Verification items for the finished model (mm, model axes). Give positions to 0.01 mm unless a question says otherwise; leave off trailing zeros. Write each loop counter-clockwise with the first axis right and the second up, starting at its lowest first coordinate (ties: lowest second). Pieces come first, ordered by that corner, then holes. Notation, with made-up numbers: M -15,-1.5 L 10,-1.5 A29 cw 10,21.5 Z; hole C 81.25,31.5 d5. An arc over 180 degrees is marked long. Answer as a JSON object with one key per item and string values.
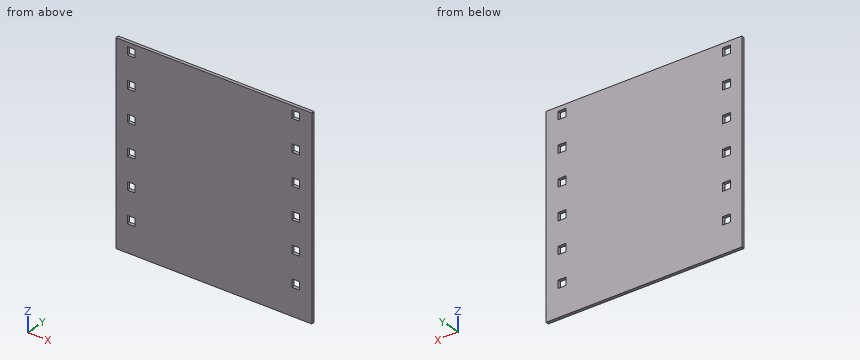
Autodesk Inventor part; units mm, degrees
ref_plane "YZ Plane" through (0, 0, 0) normal (1, 0, 0) x (0, 1, 0)
ref_plane "XZ Plane" through (0, 0, 0) normal (0, 1, 0) x (-1, 0, 0)
ref_plane "XY Plane" through (0, 0, 0) normal (0, 0, 1) x (1, 0, 0)
sketch "Эскиз1" plane through (0, 0, 0) normal (0, 1, 0) x (-1, 0, 0)
  line L0 (125, 125) -> (-125, 125)
  line L1 (-125, 125) -> (-125, -125)
  line L2 (-125, -125) -> (125, -125)
  line L3 (125, -125) -> (125, 125)
  line L4 (125, 125) -> (-125, -125) construction
  line L5 (-125, 125) -> (125, -125) construction
  point P0 (0, 0)
  dimension "d0" = 250
  dimension "d1" = 250
extrude "Выдавливание1" add sketch "Эскиз1" along normal blind 4
sketch "Эскиз2" plane through (0, 0, 0) normal (0, -1, 0) x (1, 0, 0)
  line L0 (-110.387511, 109.588885) -> (-110.387511, 119.588885)
  line L1 (-100.387511, 109.588885) -> (-110.387511, 109.588885)
  line L2 (-100.387511, 119.588885) -> (-100.387511, 109.588885)
  line L3 (-110.387511, 119.588885) -> (-100.387511, 119.588885)
  line L4 (-110.387511, 29.588885) -> (-110.387511, 39.588885)
  line L5 (-100.387511, 29.588885) -> (-110.387511, 29.588885)
  line L6 (-100.387511, 39.588885) -> (-100.387511, 29.588885)
  line L7 (-110.387511, 39.588885) -> (-100.387511, 39.588885)
  line L8 (-110.387511, -10.411115) -> (-110.387511, -0.411115)
  line L9 (-100.387511, -10.411115) -> (-110.387511, -10.411115)
  line L10 (-100.387511, -0.411115) -> (-100.387511, -10.411115)
  line L11 (-110.387511, -0.411115) -> (-100.387511, -0.411115)
  line L12 (125, 125) -> (125, -125)
  line L13 (-125, 125) -> (125, 125)
  line L14 (-125, -125) -> (-125, 125)
  line L15 (125, -125) -> (-125, -125)
  line L16 (109.612489, 109.588885) -> (109.612489, 119.588885)
  line L17 (109.612489, 119.588885) -> (99.612489, 119.588885)
  line L18 (99.612489, 119.588885) -> (99.612489, 109.588885)
  line L19 (99.612489, 109.588885) -> (109.612489, 109.588885)
  line L20 (109.612489, 29.588885) -> (109.612489, 39.588885)
  line L21 (109.612489, 39.588885) -> (99.612489, 39.588885)
  line L22 (99.612489, 39.588885) -> (99.612489, 29.588885)
  line L23 (99.612489, 29.588885) -> (109.612489, 29.588885)
  line L24 (109.612489, -10.411115) -> (109.612489, -0.411115)
  line L25 (109.612489, -0.411115) -> (99.612489, -0.411115)
  line L26 (99.612489, -0.411115) -> (99.612489, -10.411115)
  line L27 (99.612489, -10.411115) -> (109.612489, -10.411115)
  line L28 (109.612488, -50.411115) -> (109.612488, -40.411115)
  line L29 (109.612488, -40.411115) -> (99.612488, -40.411115)
  line L30 (99.612488, -40.411115) -> (99.612488, -50.411115)
  line L31 (99.612488, -50.411115) -> (109.612488, -50.411115)
  line L32 (109.612488, -90.411115) -> (109.612488, -80.411115)
  line L33 (109.612488, -80.411115) -> (99.612488, -80.411115)
  line L34 (99.612488, -80.411115) -> (99.612488, -90.411115)
  line L35 (99.612488, -90.411115) -> (109.612488, -90.411115)
  line L36 (-100.387512, -80.411115) -> (-100.387512, -90.411115)
  line L37 (-110.387512, -81.025031) -> (-100.387512, -81.025031)
  line L38 (-110.387512, -90.411115) -> (-110.387512, -80.411115)
  line L39 (-100.387512, -110) -> (-110.387512, -110)
  line L40 (-100.387512, -40.411115) -> (-100.387512, -50.411115)
  line L41 (-100.387512, -50.411115) -> (-110.387512, -50.411115)
  line L42 (-110.387512, -50.411115) -> (-110.387512, -40.411115)
  line L43 (-110.387512, -40.411115) -> (-100.387512, -40.411115)
  line L44 (-100.387512, 74.588885) -> (-100.387512, 69.588885)
  line L45 (-100.387512, 79.588885) -> (-100.387512, 74.588885)
  line L46 (-110.387512, 79.588885) -> (-100.387512, 79.588885)
  line L47 (-110.387512, 74.588885) -> (-110.387512, 79.588885)
  line L48 (-110.387512, 69.588885) -> (-110.387512, 74.588885)
  line L49 (-100.387512, 69.588885) -> (-110.387512, 69.588885)
  line L50 (109.612488, 79.588885) -> (99.612488, 79.588885)
  line L51 (99.612488, 69.588885) -> (109.612488, 69.588885)
  line L52 (99.612488, 74.588885) -> (99.612488, 69.588885)
  line L53 (109.612488, 69.588885) -> (109.612488, 74.588885)
  line L54 (109.612488, 74.588885) -> (109.612488, 79.588885)
  line L55 (99.612488, 79.588885) -> (99.612488, 74.588885)
  circle A0 centre (104.612488, -65.411115) radius 2
  circle A1 centre (104.612488, -25.411115) radius 2
  circle A2 centre (104.612488, 14.588885) radius 2
  circle A3 centre (104.612488, 54.588885) radius 2
  circle A4 centre (104.612488, 94.588885) radius 2
  circle A5 centre (-105.387512, 94.588885) radius 2
  circle A6 centre (-105.387512, 54.588885) radius 2
  circle A7 centre (-105.387512, 14.588885) radius 2
  circle A8 centre (-105.387512, -25.411115) radius 2
  circle A9 centre (-105.387512, -65.411115) radius 2
  point P0 (0, 0)
sketch "Эскиз2 outline for Выдавливание2" plane through (0, 0, 0) normal (0, -1, 0) x (1, 0, 0)
  line L0 (-110.387511, -10.411115) -> (-100.387511, -10.411115)
  line L1 (-110.387511, -0.411115) -> (-110.387511, -10.411115)
  line L2 (-100.387511, -0.411115) -> (-110.387511, -0.411115)
  line L3 (-100.387511, -10.411115) -> (-100.387511, -0.411115)
  line L4 (-110.387511, 29.588885) -> (-100.387511, 29.588885)
  line L5 (-110.387511, 39.588885) -> (-110.387511, 29.588885)
  line L6 (-100.387511, 39.588885) -> (-110.387511, 39.588885)
  line L7 (-100.387511, 29.588885) -> (-100.387511, 39.588885)
  line L8 (-110.387511, 109.588885) -> (-100.387511, 109.588885)
  line L9 (-110.387511, 119.588885) -> (-110.387511, 109.588885)
  line L10 (-100.387511, 119.588885) -> (-110.387511, 119.588885)
  line L11 (-100.387511, 109.588885) -> (-100.387511, 119.588885)
  line L12 (109.612488, -90.411115) -> (109.612488, -80.411115)
  line L13 (99.612488, -90.411115) -> (109.612488, -90.411115)
  line L14 (99.612488, -80.411115) -> (99.612488, -90.411115)
  line L15 (109.612488, -80.411115) -> (99.612488, -80.411115)
  line L16 (109.612488, -50.411115) -> (109.612488, -40.411115)
  line L17 (99.612488, -50.411115) -> (109.612488, -50.411115)
  line L18 (99.612488, -40.411115) -> (99.612488, -50.411115)
  line L19 (109.612488, -40.411115) -> (99.612488, -40.411115)
  line L20 (109.612489, -10.411115) -> (109.612489, -0.411115)
  line L21 (99.612489, -10.411115) -> (109.612489, -10.411115)
  line L22 (99.612489, -0.411115) -> (99.612489, -10.411115)
  line L23 (109.612489, -0.411115) -> (99.612489, -0.411115)
  line L24 (109.612489, 29.588885) -> (109.612489, 39.588885)
  line L25 (99.612489, 29.588885) -> (109.612489, 29.588885)
  line L26 (99.612489, 39.588885) -> (99.612489, 29.588885)
  line L27 (109.612489, 39.588885) -> (99.612489, 39.588885)
  line L28 (109.612489, 109.588885) -> (109.612489, 119.588885)
  line L29 (99.612489, 109.588885) -> (109.612489, 109.588885)
  line L30 (99.612489, 119.588885) -> (99.612489, 109.588885)
  line L31 (109.612489, 119.588885) -> (99.612489, 119.588885)
  line L32 (-100.387512, -80.411115) -> (-110.387512, -80.411115)
  line L33 (-100.387512, -90.411115) -> (-100.387512, -80.411115)
  line L34 (-110.387512, -90.411115) -> (-100.387512, -90.411115)
  line L35 (-110.387512, -80.411115) -> (-110.387512, -90.411115)
  line L36 (-100.387512, -40.411115) -> (-110.387512, -40.411115)
  line L37 (-100.387512, -50.411115) -> (-100.387512, -40.411115)
  line L38 (-110.387512, -50.411115) -> (-100.387512, -50.411115)
  line L39 (-110.387512, -40.411115) -> (-110.387512, -50.411115)
  line L40 (-100.387512, 69.588885) -> (-100.387512, 79.588885)
  line L41 (-100.387512, 79.588885) -> (-110.387512, 79.588885)
  line L42 (-110.387512, 79.588885) -> (-110.387512, 69.588885)
  line L43 (-110.387512, 69.588885) -> (-100.387512, 69.588885)
  line L44 (109.612488, 79.588885) -> (99.612488, 79.588885)
  line L45 (99.612488, 79.588885) -> (99.612488, 69.588885)
  line L46 (99.612488, 69.588885) -> (109.612488, 69.588885)
  line L47 (109.612488, 69.588885) -> (109.612488, 79.588885)
extrude "Выдавливание2" cut sketch "Эскиз2 outline for Выдавливание2" against normal up to surface (4 mm away)
properties part number "Платформа подъёмника"
1) Section check A-A on z = 35.5. Record the boundary of the cut face in (x, y), and give its area (3 significant figures).
Completed:
{"outline": "M -125,0 L -110.39,0 L -110.39,4 L -125,4 Z; M -100.39,0 L 99.61,0 L 99.61,4 L -100.39,4 Z; M 109.61,0 L 125,0 L 125,4 L 109.61,4 Z", "area": "920 mm2"}
2) Section check B-B on y = 2.6. Count the separate pieces of the cut face and the enclosed holes in it, and give its area (3 significant figures).
Completed:
{"separate pieces": "1", "enclosed holes": "12", "area": "61,300 mm2"}
3) Thickness scan on L1, parallel to X at y = 1.95, z = -46.5. Record the ranges inside material, lowest first.
Completed:
{"L1": "x = -125 to -110.39, -100.39 to 99.61, 109.61 to 125"}
